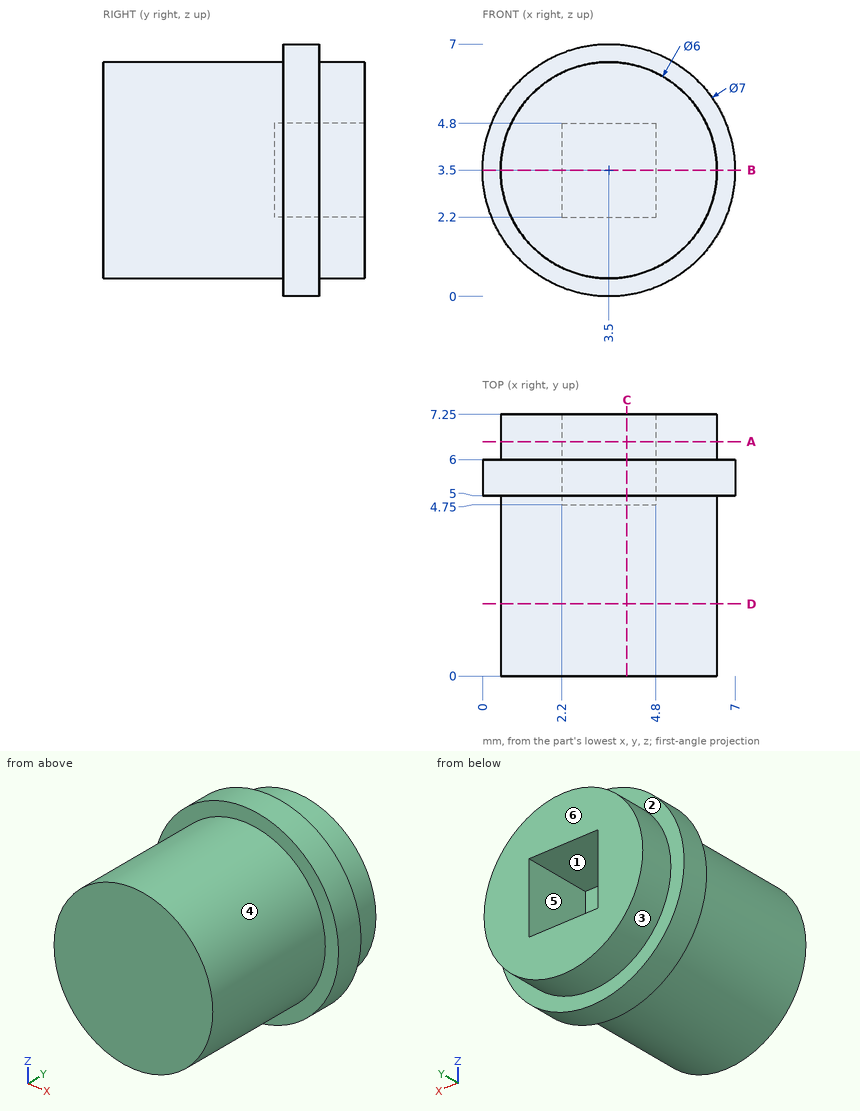
Here's the drawing with two shaded views (mm, measured from the low corner). I have some questions. A direction names the side the tool comes from. Coordinates: 2 decimals unless noted, no trailing zeros. Loops run counter-clockwise (first coordinate to the right, second up) from the corner with the lowest first, then second, coordinate; pieces in that order, holes last. Notation, with made-up numbers: (-27.75, 26.5) -> (10.25, 26.5) arc R5 cw to (10.25, 32.5) -> close; hole circle Ø2 at (75, 8). An arc over 180 degrees is marked (long way). Put each result on its own line as item: value. Start each with the question number.
Q1. I want a section at A-A (y = 6.5). Write out the boundary of the cut face in (x, z).
Q2. I want a section at D-D (y = 2). Write out the boundary of the cut face in (x, z).
Q3. Thinking about a two-plate mould opening in X: for the marked faces 1, 2 and 3, which applies, pulls with the +X half, pulls with the -X half, needs draft (parallel to the pull), parting line crosses it, or undercut?
Q4. If I drill on line 1 (X direction, y = 6.75, z = 3.5); line 2 (Y direction, x = 2.25, z = 2.25); line 3 (Y direction, x = 6.75, z = 4.5), over which ranges is the centre line in solid material (lowest first)? Write a range as [from, to].
Q5. I want a section at C-C (x = 4). Write out the boundary of the cut face in (y, z).
Q6. For the marked faces 4, 5 and 6, which set-ups out of +Z, -Z, +X, -X, +Y, -Y let a thin tool reach every point of the face, with its end or its side?
Q7. I'm going to push flat-ended pins straight in: P1, Ø0.8, axis at y = 6, z = 4, coming from the +X side; P2, Ø1.5, axis at y = 2, z = 3, coming from the -X side; P3, Ø2, axis at y = 5, z = 1.5, coming from the +X side. Where does each tip first touch, or does it pass through?
Q8. I want a section at B-B (z = 3.5). Write out the boundary of the cut face in (x, y).
Taken from the geometry:
1. outline: circle Ø6 at (3.5, 3.5); hole (2.2, 2.2) -> (4.8, 2.2) -> (4.8, 4.8) -> (2.2, 4.8) -> close
2. outline: circle Ø6 at (3.5, 3.5)
3. face 1: undercut
3. face 2: needs draft
3. face 3: parting line crosses it
4. line 1: x = [0.5, 2.2], [4.8, 6.5]
4. line 2: y = [0, 4.75]
4. line 3: y = [5, 6]
5. outline: (0, 0.54) -> (5, 0.54) -> (5, 0.04) -> (6, 0.04) -> (6, 0.54) -> (7.25, 0.54) -> (7.25, 2.2) -> (4.75, 2.2) -> (4.75, 4.8) -> (7.25, 4.8) -> (7.25, 6.46) -> (6, 6.46) -> (6, 6.96) -> (5, 6.96) -> (5, 6.46) -> (0, 6.46) -> close
6. face 4: -Y
6. face 5: +Y
6. face 6: +Z, -Z, +X, -X, +Y
7. P1: stops at x = 7
7. P2: stops at x = 0.5
7. P3: stops at x = 6.85
8. outline: (0, 5) -> (0.5, 5) -> (0.5, 0) -> (6.5, 0) -> (6.5, 5) -> (7, 5) -> (7, 6) -> (6.5, 6) -> (6.5, 7.25) -> (4.8, 7.25) -> (4.8, 4.75) -> (2.2, 4.75) -> (2.2, 7.25) -> (0.5, 7.25) -> (0.5, 6) -> (0, 6) -> close
